Source: CAD feature listing. Evaluate the final solid. Frame: model axes, mm. Round coordinates to 2 decimals unless told otherwise and drop trailing zeros. Loops run counter-clockwise (first coordinate to the right, second up) from the corner with the lowest first, then second, coordinate; pieces in that order, holes last. Notation, with made-up numbers: M -13,87 L 26,87 A27 ccw 26,107 Z; hole C 15.5,13 d5. An arc over 180 degrees is marked long. Answer as CSV lines item,"result". Start each with the question number.
```python
from build123d import *

# Parameters (mm, degrees)
SKETCH_1_W      = 90
SKETCH_1_H      = 45
SKETCH_1_R      = 4.25
EXTRUDE_1_DEPTH = 2.5
FILLET_1_R      = 1


with BuildPart() as part:
    # Эскиз1 → Бобышка-Вытянуть1 (new body)
    with BuildSketch(Plane.XY):
        Rectangle(SKETCH_1_W, SKETCH_1_H)
        with Locations((-31, 0)):
            Circle(SKETCH_1_R, mode=Mode.SUBTRACT)
        with Locations((31, 0)):
            Circle(SKETCH_1_R, mode=Mode.SUBTRACT)
    extrude(amount=EXTRUDE_1_DEPTH)

    # Скругление1
    fillet_1_edges = [part.edges().sort_by_distance(p)[0] for p in [
        (45, -22.5, 1.25),
        (-45, -22.5, 1.25),
        (-45, 22.5, 1.25),
        (45, 22.5, 1.25),
    ]]
    fillet(fillet_1_edges, radius=FILLET_1_R)


solid = part.part
```
1) Section C-C, the plane y = 0. Return loops of the section in (x, z), and give its area (4 significant figures).
2) Ray query, line 1 along Y through (x, z) = (31, 1.25); line 2 along X through (y, z) = (3, 1.3); line 3 along Y through (x, z) = (-34, 0.65). Return the intervals inside material, ascending.
3) Section A-A, the plane x = 29. Return loops of the section in (y, z), and give its area (4 significant figures).
4) Mould query, pull axis Y, two halves, no side actions, for faces 1 (the cylindrical face through (26.754, 0.187, 1.232)), 2 (the flat face through (-1, 22.5, 1)), 3 (the flat face through (-45, 0, 1)), 4 (the cylindrical face through (-35.246, 0.187, 1.232)). Classes: pulls with the +Y half, pulls with the -Y half, needs draft (parallel to the pull), parting line crosses it, or undercut.
5) Section D-D, the plane x = -31. Return loops of the section in (y, z).
6) Section B-B, the plane z = 0.6. Return loops of the section in (x, y).
Findings below:
1,outline,"M -45,0 L -35.25,0 L -35.25,2.5 L -45,2.5 Z; M -26.75,0 L 26.75,0 L 26.75,2.5 L -26.75,2.5 Z; M 35.25,0 L 45,0 L 45,2.5 L 35.25,2.5 Z"
1,area,"182.5 mm²"
2,line 1,"-22.5 to -4.25, 4.25 to 22.5"
2,line 2,"-45 to -34.01, -27.99 to 27.99, 34.01 to 45"
2,line 3,"-22.5 to -3.01, 3.01 to 22.5"
3,outline,"M -22.5,0 L -3.75,0 L -3.75,2.5 L -22.5,2.5 Z; M 3.75,0 L 22.5,0 L 22.5,2.5 L 3.75,2.5 Z"
3,area,"93.75 mm²"
4,face 1,"undercut"
4,face 2,"pulls with the +Y half"
4,face 3,"needs draft"
4,face 4,"undercut"
5,outline,"M -22.5,0 L -4.25,0 L -4.25,2.5 L -22.5,2.5 Z; M 4.25,0 L 22.5,0 L 22.5,2.5 L 4.25,2.5 Z"
6,outline,"M -45,-21.5 A1 ccw -44,-22.5 L 44,-22.5 A1 ccw 45,-21.5 L 45,21.5 A1 ccw 44,22.5 L -44,22.5 A1 ccw -45,21.5 Z; hole C -31,0 d8.5; hole C 31,0 d8.5"
